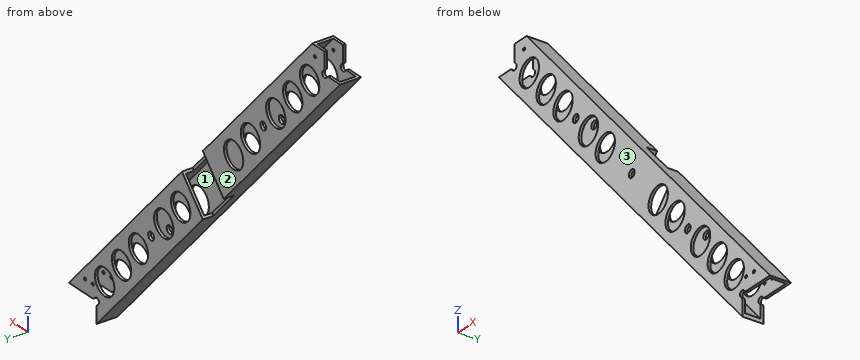
from build123d import *

# Parameters (mm, degrees)
BOSS_EXTRUDE1_DEPTH          = 25.4
CUT_EXTRUDE1_DEPTH           = 12.7
SKETCH3_W                    = 44.450000002
SKETCH3_H                    = 19.05
CUT_EXTRUDE2_DEPTH           = 645.494549375
F_3_8_0_375_DIAMETER_HOLE1_D = 9.525
CUT_EXTRUDE3_DEPTH           = 637.52463446
F_8_32_TAPPED_HOLE1_D        = 3.4544
SKETCH9_R                    = 3.81
CUT_EXTRUDE4_DEPTH           = 637.52463446
FILLET1_R                    = 3.81
F_8_32_TAPPED_HOLE2_D        = 3.4544
SKETCH12_R                   = 15.875000001
CUT_EXTRUDE5_DEPTH           = 637.52463446


with BuildPart() as part:
    # Sketch1 → Boss-Extrude1 (new body)
    with BuildSketch(Plane(origin=(0, 0, 0), x_dir=(1, 0, 0), z_dir=(0, 1, 0))):
        Polygon((386.547411153, 441.325), (432.072013268, 441.325), (12.7, -22.245579509), (12.7, 25.4), (-12.7, 25.4), (386.547411153, 466.725), align=None)
    extrude(amount=BOSS_EXTRUDE1_DEPTH)

    # Sketch2 → Cut-Extrude1 (cut)
    with BuildSketch(Plane(origin=(0, 25.4, 0), x_dir=(1, 0, 0), z_dir=(0, 1, 0))):
        Polygon((212.323705576, 274.139463524), (246.575140768, 236.278192008), (212.323705576, 198.416920491), (178.072270385, 236.278192008), align=None)
    extrude(amount=-CUT_EXTRUDE1_DEPTH, mode=Mode.SUBTRACT)

    # Sketch3 → Cut-Extrude2 (cut, through all)
    with BuildSketch(Plane(origin=(-5.351336248, 0, 5.915325694), x_dir=(-0.7415747649396567, 0, -0.6708702318665609), z_dir=(0.6708702318665609, 0, -0.7415747649396567))):
        with Locations((1.058103403, 12.7)):
            Rectangle(SKETCH3_W, SKETCH3_H)
    extrude(amount=CUT_EXTRUDE2_DEPTH, mode=Mode.SUBTRACT)

    # 3_8 _0.375_ Diameter Hole1 (through all)
    with Locations(Plane(origin=(0, 25.4, 0), x_dir=(1, 0, 0), z_dir=(0, 1, 0))):
        with Locations((113.347215967, 126.870346004), (297.173362109, 330.070346004), (205.260289038, 228.470346004)):
            Hole(F_3_8_0_375_DIAMETER_HOLE1_D / 2)

    # Sketch6 → Cut-Extrude3 (cut, through all)
    with BuildSketch(Plane(origin=(0, 25.4, 0), x_dir=(1, 0, 0), z_dir=(0, 1, 0))):
        Polygon((12.7, -22.245579509), (32.824602115, 0), (12.7, 0), align=None)
    extrude(amount=-CUT_EXTRUDE3_DEPTH, mode=Mode.SUBTRACT)

    # 8-32 Tapped Hole1 (through all)
    with Locations(Plane(origin=(0, 25.4, 0), x_dir=(1, 0, 0), z_dir=(0, 1, 0))):
        with Locations((28.575, 12.7)):
            Hole(F_8_32_TAPPED_HOLE1_D / 2)

    # Sketch9 → Cut-Extrude4 (cut, through all)
    with BuildSketch(Plane(origin=(0, 25.4, 0), x_dir=(1, 0, 0), z_dir=(0, 1, 0))):
        with Locations((12.7, 25.4)):
            Circle(SKETCH9_R)
        with Locations((386.547411153, 441.325)):
            Circle(SKETCH9_R)
    extrude(amount=-CUT_EXTRUDE4_DEPTH, mode=Mode.SUBTRACT)

    # Fillet1
    fillet1_edges = [part.edges().sort_by_distance(p)[0] for p in [
        (12.7, 1.5875, -21.59),
        (8.89, 1.5875, -25.4),
        (8.89, 23.8125, -25.4),
        (12.7, 23.8125, -21.59),
        (390.357411153, 1.5875, -441.325),
        (386.547411153, 1.5875, -445.135),
        (390.357411153, 23.8125, -441.325),
        (386.547411153, 23.8125, -445.135),
    ]]
    fillet(fillet1_edges, radius=FILLET1_R)

    # 8-32 Tapped Hole2 (through all)
    with Locations(Plane(origin=(0, 25.4, 0), x_dir=(1, 0, 0), z_dir=(0, 1, 0))):
        with Locations((392.897411153, 425.45), (405.597411153, 425.45)):
            Hole(F_8_32_TAPPED_HOLE2_D / 2)

    # Sketch12 → Cut-Extrude5 (cut, through all)
    with BuildSketch(Plane(origin=(0, 25.4, 0), x_dir=(1, 0, 0), z_dir=(0, 1, 0))):
        with Locations(Location((37.163816951, 42.657806031, 0), (0, 0, 270))):
            Circle(SKETCH12_R)
        with Locations(Location((64.853985771, 73.266304454, 0), (0, 0, 270))):
            Circle(SKETCH12_R)
        with Locations(Location((92.544154592, 103.874802877, 0), (0, 0, 270))):
            Circle(SKETCH12_R)
        with Locations(Location((134.150277343, 149.865889131, 0), (0, 0, 90))):
            Circle(SKETCH12_R)
        with Locations(Location((161.840446163, 180.474387554, 0), (0, 0, 90))):
            Circle(SKETCH12_R)
        with Locations(Location((373.356761126, 414.282885977, 0), (0, 0, 90))):
            Circle(SKETCH12_R)
        with Locations(Location((345.666592305, 383.674387554, 0), (0, 0, 90))):
            Circle(SKETCH12_R)
        with Locations(Location((317.976423485, 353.065889131, 0), (0, 0, 90))):
            Circle(SKETCH12_R)
        with Locations(Location((248.680131914, 276.466304454, 0), (0, 0, 270))):
            Circle(SKETCH12_R)
        with Locations(Location((276.370300734, 307.074802877, 0), (0, 0, 270))):
            Circle(SKETCH12_R)
    extrude(amount=-CUT_EXTRUDE5_DEPTH, mode=Mode.SUBTRACT)


solid = part.part
Could you check a few things on this model? Use its own coordinates, in mm. Face numbers are marked on the shaded views. Coordinates: 2 decimals unless noted, no trailing zeros. Loops run counter-clockwise (first coordinate to the right, second up) from the corner with the lowest first, then second, coordinate; pieces in that order, holes last.
1. We'd pull the mould along Y, two halves only. Please class the marked faces 1, 2 and 3: released by +Y, released by -Y, zero draft, split by the parting line, or undercut.
2. Imagine slicing it at C-C (z = -345). Please give me the cut outline in (x, y) (3 decimals), and give its area (3 significant figures).
3. Imagine slicing it at B-B (y = 17.25). Please give me the cut outline in (x, z) (3 decimals).
4. Imagine slicing it at D-D (z = -251.5). Please give me the cut outline in (x, y) (3 decimals).
5. Imagine slicing it at A-A (x = 340). Please give me the cut outline in (y, z) (3 decimals).
6. For P1, Ø10, axis at y = 7.5, z = -351.5, coming from the +X side; P2, Ø9, axis at x = 386.55, z = -441.32, coming from the +Y side; P3, Ø4, axis at y = 18.5, z = -277.5, coming from the -X side; P4, Ø6, axis at y = 8, z = -60.5, coming from the -X side, each with a flat end and sliding along its axis, tell me the tip position at first contact or that it passes through.
7. I need wall thicknesses on L1, parallel to X at y = 2.45, z = -425.45; L2, parallel to X at y = 4.5, z = -153; L3, parallel to Z at x = 92, y = 21.5. Which ranges of each line are inside material? Lowest first, please.
Computed values:
1. face 1: undercut
1. face 2: released by +Y
1. face 3: released by -Y
2. outline: (276.428, 0) - (304.303, 0) - (304.303, 3.175) - (280.71, 3.175) - (280.71, 22.225) - (304.303, 22.225) - (304.303, 25.4) - (276.428, 25.4) - close; (331.65, 0) - (344.931, 0) - (344.931, 25.4) - (331.65, 25.4) - (331.65, 22.225) - (340.65, 22.225) - (340.65, 3.175) - (331.65, 3.175) - close
2. area: 424 mm2
3. outline: (-12.7, -25.4) - (178.072, -236.278) - (180.213, -233.912) - (-8.419, -25.4) - close; (28.543, 0) - (210.183, -200.783) - (212.324, -198.417) - (32.825, 0) - close; (212.324, -274.139) - (386.547, -466.725) - (386.547, -461.992) - (214.464, -271.773) - close; (244.434, -238.645) - (427.791, -441.325) - (432.072, -441.325) - (246.575, -236.278) - close
4. outline: (191.843, 0) - (260.346, 0) - (260.346, 25.4) - (232.805, 25.4) - (232.805, 22.225) - (256.064, 22.225) - (256.064, 3.175) - (196.124, 3.175) - (196.124, 12.7) - (191.843, 12.7) - close
5. outline: (0, -415.272) - (25.4, -415.272) - (25.4, -398.504) - (22.225, -398.504) - (22.225, -410.539) - (3.175, -410.539) - (3.175, -398.504) - (0, -398.504) - close; (0, -368.845) - (3.175, -368.845) - (3.175, -344.282) - (22.225, -344.282) - (22.225, -368.845) - (25.4, -368.845) - (25.4, -339.549) - (0, -339.549) - close
6. P1: stops at x = 355.33
6. P2: stops at y = 25.4
6. P3: stops at x = 213.55
6. P4: stops at x = 16.34
7. L1: x = 349.21 to 362.07, 384.64 to 391.17, 394.62 to 403.87, 407.32 to 417.71
7. L2: x = 102.73 to 107.02, 166.96 to 171.24
7. L3: z = -141.13 to -136.4, -70.14 to -65.41
